from build123d import *

# Parameters (mm, degrees)
BASE_EXTRUDE_DEPTH = 355.6


with BuildPart() as part:
    # Sketch1 → Base-Extrude (new body)
    with BuildSketch(Plane.XY):
        with BuildLine():
            Line((0, 0), (34.925, 0))
            Line((34.925, 0), (34.925, 5.470090329))
            ThreePointArc((34.925, 5.470090329), (34.41915145, 6.991217504), (33.103088283, 7.906470681))
            ThreePointArc((33.103088283, 7.906470681), (31.394911277, 8.696422297), (29.987795308, 9.946189033))
            ThreePointArc((29.987795308, 9.946189033), (29.174834337, 11.354573038), (28.8925, 12.956053095))
            Line((28.8925, 12.956053095), (28.8925, 27.94))
            ThreePointArc((28.8925, 27.94), (29.319092252, 29.348938498), (30.455576923, 30.284615385))
            ThreePointArc((30.455576923, 30.284615385), (36.813334648, 42.22416693), (26.3525, 50.8))
            Line((26.3525, 50.8), (8.5725, 50.8))
            ThreePointArc((8.5725, 50.8), (-1.888334648, 42.22416693), (4.469423077, 30.284615385))
            ThreePointArc((4.469423077, 30.284615385), (5.605907748, 29.348938498), (6.0325, 27.94))
            Line((6.0325, 27.94), (6.0325, 12.956053095))
            ThreePointArc((6.0325, 12.956053095), (5.750165663, 11.354573038), (4.937204692, 9.946189033))
            ThreePointArc((4.937204692, 9.946189033), (3.530088723, 8.696422297), (1.821911717, 7.906470681))
            ThreePointArc((1.821911717, 7.906470681), (0.50584855, 6.991217504), (0, 5.470090329))
            Line((0, 5.470090329), (0, 0))
        make_face()
    extrude(amount=BASE_EXTRUDE_DEPTH)


solid = part.part
Design review of the part built by this model. Coordinates are the model's own, in mm. A direction names the side the tool comes from. Round coordinates to 2 decimals unless told otherwise and drop trailing zeros. Order: outer loops, then holes, each group sorted by start corner. A loop starts at its lowest first (then second) coordinate and runs counter-clockwise, first axis right, second up. Notation, with made-up numbers: M 57,14 L 115,14 A17 ccw 115,24 Z; hole C 9,32.25 d5. An arc over 180 degrees is marked long. Answer as CSV lines item,"result". Start each with the question number.
1) Tool access review of faces 1 (the face through (0, 3, 175)), 2 (the face through (36.852, 42.023, 175.311)), 3 (the face through (17, 26, 355.6)), 4 (the face through (34.925, 3, 175)), 5 (the face through (6.032, 21, 175)): name each direction out of +Z, -Z, +X, -X, +Y, -Y from which nothing blocks a thin tool from reaching the whole face with its end or side.
2) Add section A-A (z = 47.5). Give the boundary of the cut face in (x, y) (1 decimal), then the cut area to 3 significant figures.
3) The part is to be moulded in two halves that separate along Y. For faces 6 (the face through (18, 50.8, 175)), 7 (the face through (17, 26, 0)), 8 (the face through (28.892, 20, 175)), 9 (the face through (17, 0, 175)), say which applies: +Y half, -Y half, draft (parallel to the pull), parting line (faces both ways), or undercut.
4) Wall thickness on line 1 along Y through (x, z) = (4.5, 154.5); line 2 along X through (y, z) = (26, 201.5); line 3 along X through (y, z) = (39.5, 69): over which ranges is each line inside the solid? List them lowest first. Write a range as [from, to].
5) Add section B-B (y = 18). Give the boundary of the cut face in (x, z), then the cut area to 3 significant figures.
6) Add section C-C (y = 46). Give the boundary of the cut face in (x, z).
7) For pin 1 Ø12 at (y, z) = (31, 100) entering from +X; pin 2 Ø7.5 at (y, z) = (17.5, 228) entering from -X; pin 3 Ø12 at (y, z) = (23.5, 265) entering from +X, all flat-tipped, find the tip position at first contact; note any pin that passes through.
Resolved:
1,face 1,"+Z, -Z, -X, -Y"
1,face 2,"+Z, -Z, +X"
1,face 3,"+Z, +X, -X, +Y, -Y"
1,face 4,"+Z, -Z, +X, -Y"
1,face 5,"+Z, -Z, -X"
2,outline,"M 0,0 L 34.9,0 L 34.9,5.5 A2.5 ccw 33.1,7.9 A6.4 cw 30,9.9 A4.7 cw 28.9,13 L 28.9,27.9 A2.5 cw 30.5,30.3 A10.7 ccw 26.4,50.8 L 8.6,50.8 A10.7 ccw 4.5,30.3 A2.5 cw 6,27.9 L 6,13 A4.7 cw 4.9,9.9 A6.4 cw 1.8,7.9 A2.5 ccw 0,5.5 Z"
2,area,"1,520 mm^2"
3,face 6,"+Y half"
3,face 7,"draft"
3,face 8,"undercut"
3,face 9,"-Y half"
4,line 1,"[0, 9.47], [30.27, 49.99]"
4,line 2,"[6.03, 28.89]"
4,line 3,"[-2.08, 37]"
5,outline,"M 6.03,0 L 28.89,0 L 28.89,355.6 L 6.03,355.6 Z"
5,area,"8,130 mm^2"
6,outline,"M -0.34,0 L 35.26,0 L 35.26,355.6 L -0.34,355.6 Z"
7,pin 1,"x = 36.55"
7,pin 2,"x = 6.03"
7,pin 3,"x = 29.43"
